Geometry: final body of the model. Coordinates: model frame, mm. A direction names the side the tool comes from. Round coordinates to 2 decimals unless told otherwise and drop trailing zeros. Loops run counter-clockwise (first coordinate to the right, second up) from the corner with the lowest first, then second, coordinate; pieces in that order, holes last. Notation, with made-up numbers: M -5.5,41 L 16.5,41 A28 ccw 16.5,69 Z; hole C 81,19.5 d6. An arc over 180 degrees is marked long. Answer as a JSON object with one key per item and string values.
from build123d import *

# Parameters (mm, degrees)
BOSS_EXTRUDE1_DEPTH      = 20
CUT_EXTRUDE1_DEPTH       = 11
SKETCH4_R                = 10
CUT_EXTRUDE2_DEPTH       = 11
BOSS_EXTRUDE2_DEPTH      = 95
BOSS_EXTRUDE2_DEPTH_BACK = 95
SKETCH6_R                = 40
CUT_EXTRUDE3_DEPTH       = 196.258176901
CUT_EXTRUDE4_DEPTH       = 108.806733567
FILLET1_R                = 1


with BuildPart() as part:
    # Sketch1 → Boss-Extrude1 (new body)
    with BuildSketch(Plane.XY):
        Polygon((10, -17.320508076), (20, 0), (10, 17.320508076), (-10, 17.320508076), (-20, 0), (-10, -17.320508076), align=None)
    extrude(amount=BOSS_EXTRUDE1_DEPTH)

    # Sketch3 → Cut-Extrude1 (cut)
    with BuildSketch(Plane(origin=(0, 0, 0), x_dir=(-1, 0, 0), z_dir=(0, 0, -1))):
        with BuildLine():
            Line((4.358898944, 9), (-4.358898944, 9))
            ThreePointArc((-4.358898944, 9), (-10, 0), (-4.358898944, -9))
            Line((-4.358898944, -9), (4.358898944, -9))
            ThreePointArc((4.358898944, -9), (8.473163206, -5.310885546), (10, 0))
            ThreePointArc((10, 0), (8.473163206, 5.310885546), (4.358898944, 9))
        make_face()
    extrude(amount=-CUT_EXTRUDE1_DEPTH, mode=Mode.SUBTRACT)

    # Sketch4 → Cut-Extrude2 (cut)
    with BuildSketch(Plane(origin=(0, 0, 11), x_dir=(-1, 0, 0), z_dir=(0, 0, -1))):
        with Locations(Location((0, 0, 0), (0, 0, 64.158067237))):
            Circle(SKETCH4_R)
    extrude(amount=-CUT_EXTRUDE2_DEPTH, mode=Mode.SUBTRACT)

    # Sketch5 → Boss-Extrude2 (add, two sides: drawn at the far end of the back side and taken through both)
    with BuildSketch(Plane(origin=(0, 0, 0), x_dir=(0, 0, -1), z_dir=(1, 0, 0)).offset(-BOSS_EXTRUDE2_DEPTH_BACK)):
        with BuildLine():
            Line((20.478916174, 40.079541402), (20.478916174, 36.84249773))
            ThreePointArc((20.478916174, 36.84249773), (-3.944487245, 0), (20.478916174, -36.84249773))
            Line((20.478916174, -36.84249773), (20.478916174, -40.079541402))
            ThreePointArc((20.478916174, -40.079541402), (-6.944487245, 0), (20.478916174, 40.079541402))
        make_face()
    extrude(amount=BOSS_EXTRUDE2_DEPTH + BOSS_EXTRUDE2_DEPTH_BACK)

    # Sketch6 → Cut-Extrude3 (cut, through all)
    with BuildSketch(Plane(origin=(95, 0, 0), x_dir=(0, 0, -1), z_dir=(1, 0, 0))):
        with Locations((36.055512755, 0)):
            Circle(SKETCH6_R)
    extrude(amount=-CUT_EXTRUDE3_DEPTH, mode=Mode.SUBTRACT)

    # Sketch7 → Cut-Extrude4 (cut, through all)
    with BuildSketch(Plane.XY.offset(11)):
        with BuildLine():
            Line((-4.358898944, 9), (4.358898944, 9))
            ThreePointArc((4.358898944, 9), (10, 0), (4.358898944, -9))
            Line((4.358898944, -9), (-4.358898944, -9))
            ThreePointArc((-4.358898944, -9), (-10, 0), (-4.358898944, 9))
        make_face()
    extrude(amount=-CUT_EXTRUDE4_DEPTH, mode=Mode.SUBTRACT)

    # Fillet1
    fillet1_edges = [part.edges().sort_by_distance(p)[0] for p in [
        (-95, 0, 3.944487245),
        (-95, 0, 6.944487245),
        (95, 0, 3.944487245),
        (95, 0, 6.944487245),
    ]]
    fillet(fillet1_edges, radius=FILLET1_R)


solid = part.part
1) Section query B-B (x = 53.5). Return the cut outline in (y, z), and give its area (3 significant figures).
Results:
{"outline": "M -40.08,-20.48 L -36.84,-20.48 A40 cw 36.84,-20.48 L 40.08,-20.48 A43 ccw Z", "area": "295 mm2"}
2) Pin query (flat end, axial travel): P1, Ø8.5, axis at x = -1, z = 9, coming from the -Y side; P2, Ø12, axis at x = 76, z = -13, coming from the -Y side; P3, Ø0.5, axis at x = -1.5, y = -9.5, coming from the +Z side; P4, Ø1, axis at x = 49, z = 8, coming from the -Y side. Return the tip coordinate at first contact, or that it passes through.
Results:
{"P1": "y = -17.32", "P2": "y = -39.47", "P3": "z = 11", "P4": "through"}
3) Ray query, line 1 (Y direction, x = 0, z = 16); line 2 (X direction, y = 0, z = 14); line 3 (X direction, y = -5.5, z = 4.5). Return the intervals inside material, ascending.
Results:
{"line 1": "-17.32 to -10, 10 to 17.32", "line 2": "-20 to -10, 10 to 20", "line 3": "-95 to -8.35, 8.35 to 95"}
4) Pull-direction query (Y, two-part tool) for faces 6 (the flat face through (-15.07, -8.54, 13.39)), 7 (the flat face through (0, -9, 7)), 8 (the flat face through (15.07, 8.54, 13.39)), 9 (the flat face through (-1, 38, -20.479)); classes: +Y half, -Y half, draft (parallel to the pull), parting line (faces both ways), or undercut.
Results:
{"face 6": "-Y half", "face 7": "undercut", "face 8": "+Y half", "face 9": "draft"}
5) Reachability of faces 1 (the cylindrical face through (-1.316, 21.238, 1.333)), 2 (the flat face through (0, 9, 7)), 3 (the flat face through (0, -17.321, 12)), 4 (the flat face through (14.93, -8.78, 13.39)), 5 (the flat face through (-14.93, 8.78, 13.39)) from +Z, -Z, +X, -X, +Y, -Y: full face, straight path, thin tool, end or side. Return the list, or none.
Results:
{"face 1": "+Z", "face 2": "+Z, -Z", "face 3": "+Z, +X, -X, -Y", "face 4": "+Z, +X, -Y", "face 5": "+Z, -X, +Y"}
6) Section query A-A (x = 0). Return the cut outline in (y, z), and give its area (3 significant figures).
Results:
{"outline": "M -40.08,-20.48 L -36.84,-20.48 A40 cw -9,2.92 L -9,11 L -10,11 L -10,20 L -17.32,20 L -17.32,3.3 A43 ccw Z; M 9,2.92 A40 cw 36.84,-20.48 L 40.08,-20.48 A43 ccw 17.32,3.3 L 17.32,20 L 10,20 L 10,11 L 9,11 Z", "area": "476 mm2"}
